Check sheet for the modelled part. Datum: model origin and axes. Units: mm. Coordinates: 2 decimals unless noted, no trailing zeros. Loops run counter-clockwise (first coordinate to the right, second up) from the corner with the lowest first, then second, coordinate; pieces in that order, holes last. Notation, with made-up numbers: (-9.5, 83) - (-0.5, 83) arc R15 ccw to (-0.5, 100) - close; hole circle Ø3 at (25, -1.5). An arc over 180 degrees is marked (long way). Write each question's results on one line, items separated by ' | '. Start each with the question number.
1. Thickness scan on line 1 (Y direction, x = 0, z = 4); line 2 (X direction, y = 8, z = 7.25); line 3 (Y direction, x = 2, z = 7). Record the ranges inside material, lowest first. Write a range as [from, to].
2. Cross-section at A-A (z = 6). Record the cut outline in (x, y).
3. Gauge pin test, flat ends, axial feed: P1, Ø2, axis at x = 2.5, z = 4.5, coming from the +Y side; P2, Ø2.5, axis at x = 8, y = 0, coming from the -Z side. Record the tip position at first contact, or that the pin passes through.
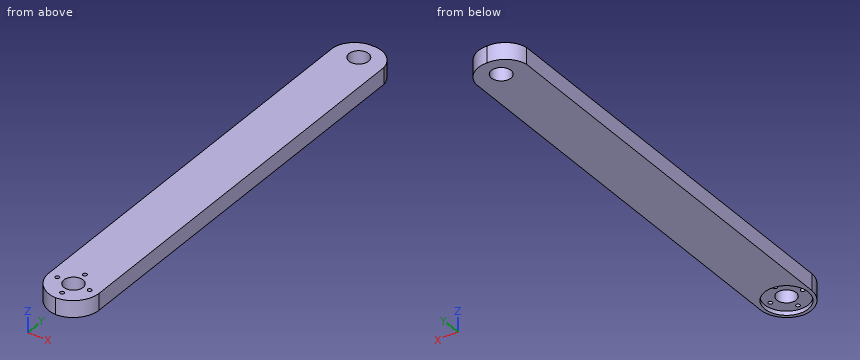
Autodesk Inventor part; units mm, degrees
ref_plane "YZ Plane" through (0, 0, 0) normal (1, 0, 0) x (0, 1, 0)
ref_plane "XZ Plane" through (0, 0, 0) normal (0, 1, 0) x (-1, 0, 0)
ref_plane "XY Plane" through (0, 0, 0) normal (0, 0, 1) x (1, 0, 0)
sketch "Sketch1" plane through (0, 0, 0) normal (0, 0, 1) x (1, 0, 0)
  arc A0 (10.5, 0) -> (0, -10.5) centre (0, 0) ccw
  circle A1 centre (0, 8) radius 0.5
  circle A2 centre (-8, 0) radius 0.5
  circle A3 centre (0, -8) radius 0.5
  circle A4 centre (8, 0) radius 0.5
  line L0 (-10.5, 0) -> (-12.5, 0) construction
  arc A5 (0, -10.5) -> (10.5, 0) centre (0, 0) ccw
  line L1 (10.5, 0) -> (12.5, 0)
  line L2 (0, -10.5) -> (0, -12.5) construction
  arc A6 (-12.5, 0) -> (0, -12.5) centre (0.4907, 0.4907) ccw
  arc A7 (0, -12.5) -> (12.5, 0) centre (-0.4907, 0.4907) ccw
  line L3 (-12.5, 0) -> (12.5, 0) construction
  line L4 (12.5, 0) -> (12.5, 200)
  line L5 (12.5, 200) -> (-12.5, 200) construction
  line L6 (-12.5, 200) -> (-12.5, 0)
  arc A8 (4.85, 200) -> (-4.85, 200) centre (0, 200) ccw
  line L7 (0, 200) -> (0, 210) construction
  arc A9 (0, 210) -> (-12.5, 200) centre (-0.6647, 198.0184) ccw
  arc A10 (12.5, 200) -> (0, 210) centre (0.6647, 198.0184) ccw
  arc A11 (-4.85, 200) -> (4.85, 200) centre (0, 200) ccw
  dimension "d0" = 21
  dimension "d1" = 1
  dimension "d2" = 1
  dimension "d3" = 1
  dimension "d4" = 1
  dimension "d5" = 8
  dimension "d6" = 8
  dimension "d7" = 8
  dimension "d8" = 8
  dimension "d14" = 12.5
  dimension "d15" = 12.5
  dimension "d16" = 12.5
  dimension "d17" = 2
  dimension "d18" = 2
  dimension "d19" = 2
  dimension "d20" = 13
  dimension "d21" = 13
  dimension "d30" = 200
  dimension "d31" = 9.7
  dimension "d32" = 12.5
  dimension "d34" = 2.5
  dimension "d35" = 2.5
  dimension "d36" = 2.5
  dimension "d37" = 10
  dimension "d38" = 12
  dimension "d39" = 12
sketch "Sketch2" plane through (0, 0, 0) normal (0, 0, 1) x (1, 0, 0)
  arc A0 (10.5, 0) -> (0, -10.5) centre (0, 0) ccw
  circle A1 centre (-8, 0) radius 0.5
  circle A2 centre (0, -8) radius 0.5
  circle A3 centre (8, 0) radius 0.5
  circle A4 centre (0, 8) radius 0.5
  arc A5 (0, -10.5) -> (10.5, 0) centre (0, 0) ccw
sketch "Sketch3" plane through (0, 0, 0) normal (0, 0, 1) x (1, 0, 0)
  arc A0 (0, 210) -> (-12.5, 200) centre (-0.6647, 198.0184) ccw
  line L0 (-12.5, 200) -> (-12.5, 0)
  arc A1 (-12.5, 0) -> (0, -12.5) centre (0.4907, 0.4907) ccw
  arc A2 (0, -12.5) -> (12.5, 0) centre (-0.4907, 0.4907) ccw
  line L1 (12.5, 0) -> (12.5, 200)
  arc A3 (12.5, 200) -> (0, 210) centre (0.6647, 198.0184) ccw
  point P0 (0, 0)
extrude "Extrusion1" add sketch "Sketch3" along normal blind 8.2
extrude "Extrusion2" cut sketch "Sketch1" along normal blind 10 contours A11 A8
extrude "Extrusion3" cut sketch "Sketch2" along normal blind 2
sketch "Sketch4" plane through (8, 0, 0) normal (0, 0, -1) x (-1, 0, 0)
  circle A0 centre (0, 0) radius 0.5
  circle A1 centre (8, 8) radius 0.5
  circle A2 centre (16, 0) radius 0.5
  circle A3 centre (8, -8) radius 0.5
  point P0 (8, 0)
hole "Hole1" at (0, 8, 0) at (8, 0, 0) at (0, -8, 0) at (-8, 0, 0) direction (0, 0, 1) diameter 2 depth 10 tip angle 118
sketch "Sketch5" plane through (0, 0, 8.2) normal (0, 0, 1) x (1, 0, 0)
  point P0 (0, 0)
sketch "Sketch6" plane through (0, 0, 8.2) normal (0, 0, 1) x (1, 0, 0)
  circle A0 centre (0, 200) radius 4.85
  point P0 (0, 0)
sketch "Sketch7" plane through (0, 0, 8.2) normal (0, 0, 1) x (1, 0, 0)
  point P0 (0, 0)
sketch "Sketch9" plane through (0, 0, 0) normal (0, 0, -1) x (-1, 0, 0)
  circle A0 centre (0, 0) radius 10.75
  dimension "d55" = 21.5
extrude "Extrusion5" cut sketch "Sketch9" against normal blind 2
sketch "Sketch10" plane through (0, 0, 2) normal (0, 0, -1) x (-1, 0, 0)
  circle A0 centre (0, 0) radius 4.75
  dimension "d58" = 9.5
extrude "Extrusion6" cut sketch "Sketch10" against normal blind 10
properties part number "BB-8_headslider_rod"
Established:
1) line 1: [-12.5, -9], [-7, -4.75], [4.75, 7], [9, 195.15], [204.85, 210] | line 2: [-12.5, -1], [1, 12.5] | line 3: [-12.27, -4.31], [4.31, 195.58], [204.42, 209.94]
2) outline: (-12.5, 0) arc R13 ccw to (0, -12.5) arc R13 ccw to (12.5, 0) - (12.5, 200) arc R12 ccw to (0, 210) arc R12 ccw to (-12.5, 200) - close; hole circle Ø2 at (-8, 0); hole circle Ø9.7 at (0, 200); hole circle Ø9.5 at (0, 0); hole circle Ø2 at (0, -8); hole circle Ø2 at (0, 8); hole circle Ø2 at (8, 0)
3) P1: y = 209.99 | P2: z = 2
